Here's how the part is built. I have some questions about the finished solid (model axes, mm). A direction names the side the tool comes from. Round coordinates to 2 decimals unless told otherwise and drop trailing zeros. Order: outer loops, then holes, each group sorted by start corner. A loop starts at its lowest first (then second) coordinate and runs counter-clockwise, first axis right, second up. Notation, with made-up numbers: (89.25, -12) -> (140.25, -12) arc R15 ccw to (140.25, 14) -> close; hole circle Ø3 at (46, 89.25). An arc over 180 degrees is marked (long way). Use a Markdown table: item, result. Add a question column.
(1) If I drill on probe 1 along Y at (x, z) = (80, 15.5); probe 2 along X at (y, z) = (40, 21.5); probe 3 along Y at (x, z) = (71, 12.5), over which ranges is the centre line in solid material (lowest first)?
(2) I want a section at C-C, the plane x = 40. Please give me the cut outline in (y, z).
(3) On a 3-axis mill with a long thin cutter (end or side, diameter ignored), from which of +Z, -Z, +X, -X, +Y, -Y can I reach the whole of each face in a straight line? I mean faces 1 (the face through (60, 24, 30)), 2 (the face through (60, 35, 15)). Say none if no direction works.
(4) I'm going to push flat-ended pins straight in: P1, Ø8, axis at y = 36.5, z = 16.5, coming from the -X side; P2, Ø16, axis at x = 80, y = 40, coming from the -Z side; P3, Ø3, axis at x = 39, z = 5, coming from the -Y side; P4, Ø1.5, axis at x = 12, z = 23, coming from the +Y side. Where does each tip first touch, or does it pass through?
(5) I want a section at D-D, the plane y = 53. Please give me the cut outline in (x, z).
(6) Thinking about a two-plate mould opening in X: for faces 3 (the face through (0, 15, 15)), 4 (the face through (30, 30, 15)), 5 (the face through (70.085, 41.302, 14.79)), which applies, pulls with the +X half, pulls with the -X half, needs draft (parallel to the pull), parting line crosses it, or undercut?
(7) I want a section at A-A, the plane x = 80. Please give me the cut outline in (y, z).
(8) I want a section at B-B, the plane z = 21.5. Please give me the cut outline in (x, y).
Autodesk Inventor part; units mm, degrees
ref_plane "YZ Plane" through (0, 0, 0) normal (1, 0, 0) x (0, 1, 0)
ref_plane "XZ Plane" through (0, 0, 0) normal (0, 1, 0) x (-1, 0, 0)
ref_plane "XY Plane" through (0, 0, 0) normal (0, 0, 1) x (1, 0, 0)
sketch "Esboço1" plane through (0, 0, 0) normal (0, 0, 1) x (1, 0, 0)
  line L0 (0, 0) -> (100, 0)
  line L1 (100, 0) -> (100, 40)
  line L2 (60, 40) -> (60, 30)
  line L3 (60, 30) -> (0, 30)
  line L4 (0, 30) -> (0, 0)
  arc A0 (100, 40) -> (60, 40) centre (80, 40) ccw
  dimension "d0" = 100
  dimension "d3" = 40
  dimension "d4" = 30
  dimension "d5" = 20
extrude "Extrusão1" add sketch "Esboço1" along normal blind 30
sketch "Esboço2" plane through (0, 0, 30) normal (0, 0, 1) x (1, 0, 0)
  arc A0 (100, 40) -> (60, 40) centre (80, 40) ccw
  point P0 (0, 0)
hole "Furo1" at (80, 40, 30) direction (0, 0, -1) diameter 20 end through all
Taken from the geometry:
| question | item | result |
|---|---|---|
| 1 | probe 1 | y = 0 to 30, 50 to 60 |
| 1 | probe 2 | x = 60 to 70, 90 to 100 |
| 1 | probe 3 | y = 0 to 35.64, 44.36 to 57.86 |
| 2 | outline | (0, 0) -> (30, 0) -> (30, 30) -> (0, 30) -> close |
| 3 | face 1 | +Z, +X, -X, +Y, -Y |
| 3 | face 2 | +Z, -Z, -X, +Y |
| 4 | P1 | stops at x = 60 |
| 4 | P2 | passes through |
| 4 | P3 | stops at y = 0 |
| 4 | P4 | stops at y = 30 |
| 5 | outline | (64.8, 0) -> (95.2, 0) -> (95.2, 30) -> (64.8, 30) -> close |
| 6 | face 3 | pulls with the -X half |
| 6 | face 4 | needs draft |
| 6 | face 5 | undercut |
| 7 | outline | (0, 0) -> (30, 0) -> (30, 30) -> (0, 30) -> close; (50, 0) -> (60, 0) -> (60, 30) -> (50, 30) -> close |
| 8 | outline | (0, 0) -> (100, 0) -> (100, 40) arc R20 ccw to (60, 40) -> (60, 30) -> (0, 30) -> close; hole circle Ø20 at (80, 40) |
